from build123d import *

# Parameters (mm, degrees)
SKETCH_1_R      = 2
SKETCH_1_R_2    = 3
EXTRUDE_1_DEPTH = 4
CHAMFER_1_SIZE  = 2


with BuildPart() as part:
    # 草图1 → 凸台-拉伸1 (new body)
    with BuildSketch(Plane.XY):
        with BuildLine():
            Line((13, 9.5), (13, -9.5))
            ThreePointArc((13, -9.5), (16.094355016, -14.122609349), (21.547406878, -13.023620928))
            Line((21.547406878, -13.023620928), (34.256888253, -0.228345114))
            ThreePointArc((34.256888253, -0.228345114), (35.858751307, 5.294230708), (32.07954512, 9.628098444))
            Line((32.07954512, 9.628098444), (19.732954267, 14.190082037))
            ThreePointArc((19.732954267, 14.190082037), (15.142096164, 13.602729051), (13, 9.5))
        make_face()
        with Locations((18, 9.5)):
            Circle(SKETCH_1_R, mode=Mode.SUBTRACT)
        with Locations((18, -9.5)):
            Circle(SKETCH_1_R, mode=Mode.SUBTRACT)
        with Locations((30, 4)):
            Circle(SKETCH_1_R_2, mode=Mode.SUBTRACT)
    extrude(amount=EXTRUDE_1_DEPTH)

    # 倒角1
    chamfer_1_edges = [part.edges().sort_by_distance(p)[0] for p in [
        (16, 9.5, 4),
        (16, -9.5, 4),
    ]]
    chamfer(chamfer_1_edges, length=CHAMFER_1_SIZE)


solid = part.part
Input: part model. Units: mm. Frame: model coordinates. Give positions to 0.01 mm unless a question says otherwise; leave off trailing zeros. Loops run counter-clockwise (first coordinate to the right, second up) from the corner with the lowest first, then second, coordinate; pieces in that order, holes last. Notation, with made-up numbers: M 39.5,22 L 58.5,22 A20 cw 58.5,58 Z; hole C 48,19.5 d4. An arc over 180 degrees is marked long. Use CSV: the item, a comma, the result in double quotes.
(1) Pin query (flat end, axial travel): P1, Ø2, axis at x = 29, z = 2.5, coming from the -Y side; P2, Ø1, axis at x = 27.5, z = 2, coming from the -Y side; P3, Ø4.5, axis at x = 18, y = 9.5, coming from the +Z side. Return the tip coordinate at first contact, or that it passes through.
Outcome:
P1,"stops at y = -6.53"
P2,"stops at y = -7.53"
P3,"stops at z = 2.25"
(2) Section C-C, the plane z = 2.7. Return loops of the section in (x, y).
Outcome:
outline,"M 13,-9.5 A5 ccw 21.55,-13.02 L 34.26,-0.23 A6 ccw 32.08,9.63 L 19.73,14.19 A5 ccw 13,9.5 Z; hole C 18,-9.5 d5.4; hole C 18,9.5 d5.4; hole C 30,4 d6"
(3) Section B-B, the plane x = 18. Return loops of the section in (y, z), plus the area to 3 significant figures.
Outcome:
outline,"M -14.5,0 L -11.5,0 L -11.5,2 L -13.5,4 L -14.5,4 Z; M -7.5,0 L 7.5,0 L 7.5,2 L 5.5,4 L -5.5,4 L -7.5,2 Z; M 11.5,0 L 14.5,0 L 14.5,4 L 13.5,4 L 11.5,2 Z"
area,"76.0 mm²"
(4) Pull-direction query (Y, two-part tool) for faces 1 (the face through (27.81, -6.72, 1.97)), 2 (the face through (16.526, -8.148, 0.986)), 3 (the face through (22, 0, 0)); classes: pulls with the +Y half, pulls with the -Y half, needs draft (parallel to the pull), parting line crosses it, or undercut.
Outcome:
face 1,"pulls with the -Y half"
face 2,"undercut"
face 3,"needs draft"
(5) Section D-D, the plane x = 28.25. Return loops of the section in (y, z), plus the area to 3 significant figures.
Outcome:
outline,"M -6.28,0 L 1.56,0 L 1.56,4 L -6.28,4 Z; M 6.44,0 L 11.04,0 L 11.04,4 L 6.44,4 Z"
area,"49.8 mm²"
(6) Section A-A, the plane y = 4. Return loops of the section in (x, z).
Outcome:
outline,"M 13,0 L 27,0 L 27,4 L 13,4 Z; M 33,0 L 36,0 L 36,4 L 33,4 Z"
(7) Material intervals for L1, parallel to Y at x = 18, z = 1; L2, parallel to Y at x = 20.75, z = 3.8; L3, parallel to Y at x = 32.25, z = 0.55, sorted ascending. Write a range as [from, to].
Outcome:
L1,"y = [-14.5, -11.5], [-7.5, 7.5], [11.5, 14.5]"
L2,"y = [-13.68, -12.12], [-6.88, 6.88], [12.12, 13.81]"
L3,"y = [-2.25, 2.02], [5.98, 9.56]"
